```python
from build123d import *

# Parameters (mm, degrees)
F0_R          = 34.544
F0_R_2        = 30.1625
F1_DEPTH      = 39.6875
F1_DEPTH_BACK = 39.6875
F0_R_3        = 28.575
F2_DEPTH      = 2.38125
F2_DEPTH_BACK = 2.38125
F3_R          = 2.54


# Not quite as in the source:
# - a length typed as a fraction of an inch, garbled in the dataset ("3 / 203.2 mm" for 3/8 in), is restored


with BuildPart() as f1:
    # F0 (on Top) → F1 (new body, two sides)
    with BuildSketch(Plane.XY) as f1_sk:
        Circle(F0_R)
        Circle(F0_R_2, mode=Mode.SUBTRACT)
    extrude(amount=F1_DEPTH)
    extrude(f1_sk.sketch, amount=-F1_DEPTH_BACK)

    # F0 (on Top) → F2 (join, two sides)
    with BuildSketch(Plane.XY) as f2_sk:
        Circle(F0_R_2)
        Circle(F0_R_3, mode=Mode.SUBTRACT)
    extrude(amount=F2_DEPTH)
    extrude(f2_sk.sketch, amount=-F2_DEPTH_BACK)

    # F3
    f3_edges = [f1.edges().sort_by_distance(p)[0] for p in [
        (-30.1625, 0, 39.6875),
        (-30.1625, 0, -39.6875),
    ]]
    fillet(f3_edges, radius=F3_R)


solid = f1.part
```
CAD build for the part. Positions are in the model's coordinates, mm. A direction names the side the tool comes from. Coordinates: 2 decimals unless noted, no trailing zeros. Order: outer loops, then holes, each group sorted by start corner. A loop starts at its lowest first (then second) coordinate and runs counter-clockwise, first axis right, second up. Notation, with made-up numbers: (-38, -34.75) - (-3, -34.75) arc R21 ccw to (-3, -26.75) - close; hole circle Ø10 at (9.5, 16.5). An arc over 180 degrees is marked (long way). Use a Markdown table: item, result. Add a question column.
(1) Saw through at C-C (z = 8). Give the cut face in (x, y) (1 decimal).
(2) Which spindle directions (+Z, -Z, +X, -X, +Y, -Y) get a long thin tool onto all of the face, cutting with end or side? Do faces 1 (the face through (27, -11, 2.381)), 2 (the face through (13, -31, 39.688)), 3 (the face through (27, -11, -2.381)). Say none if no direction does.
(3) Saw through at A-A (x = 0). Give the cut face in (y, z) (1 decimal), then the cut area to 3 significant figures.
(4) Flat gauge pins, fed straight in: pin 1 (3 mm diameter, centred on y = -22, z = 28, fed in from +X); pin 2 (3 mm diameter, centred on x = 1, z = 21.5, fed in from +Y); pin 3 (12 mm diameter, centred on y = -25.5, z = 7.5, fed in from -X); pin 4 (3 mm diameter, centred on x = 24, y = 27, fed in from +Z). Where does each tip first touch, or does it go through?
(5) Pull direction X, two halves, no side cores. Call faces 4 (the face through (13, -31, -39.688)), 5 (the face through (-30.133, 1.326, -19.521)), 6 (the face through (-4.5, 34.25, 0.56)): +X half, -X half, draft (parallel to the pull), parting line (faces both ways), or undercut.
(6) Drill centre lines: line 1 along Y through (x, z) = (0, -24.5); line 2 along Y through (x, z) = (0, -1) (3 decimals); line 3 along X through (y, z) = (-1, -21). Where is each one in solid material? Low to high. Write a range as [from, to].
Solved:
| question | item | result |
|---|---|---|
| 1 | outline | circle Ø69.1 at (0, 0); hole circle Ø60.3 at (0, 0) |
| 2 | face 1 | +Z |
| 2 | face 2 | +Z, +X, -X, +Y, -Y |
| 2 | face 3 | -Z |
| 3 | outline | (-34.5, -39.7) - (-32.7, -39.7) arc R2.5 ccw to (-30.2, -37.1) - (-30.2, -2.4) - (-28.6, -2.4) - (-28.6, 2.4) - (-30.2, 2.4) - (-30.2, 37.1) arc R2.5 ccw to (-32.7, 39.7) - (-34.5, 39.7) - close; (28.6, -2.4) - (30.2, -2.4) - (30.2, -37.1) arc R2.5 ccw to (32.7, -39.7) - (34.5, -39.7) - (34.5, 39.7) - (32.7, 39.7) arc R2.5 ccw to (30.2, 37.1) - (30.2, 2.4) - (28.6, 2.4) - close |
| 3 | area | 705 mm² |
| 4 | pin 1 | stops at x = 27.8 |
| 4 | pin 2 | stops at y = 34.54 |
| 4 | pin 3 | stops at x = -28.51 |
| 4 | pin 4 | passes through |
| 5 | face 4 | draft |
| 5 | face 5 | undercut |
| 5 | face 6 | parting line |
| 6 | line 1 | y = [-34.54, -30.16], [30.16, 34.54] |
| 6 | line 2 | y = [-34.544, -28.575], [28.575, 34.544] |
| 6 | line 3 | x = [-34.53, -30.15], [30.15, 34.53] |
